Autodesk Inventor part; units mm, degrees
ref_plane "YZ Plane" through (0, 0, 0) normal (1, 0, 0) x (0, 1, 0)
ref_plane "XZ Plane" through (0, 0, 0) normal (0, 1, 0) x (-1, 0, 0)
ref_plane "XY Plane" through (0, 0, 0) normal (0, 0, 1) x (1, 0, 0)
sketch "Sketch1" plane through (0, 0, 0) normal (1, 0, 0) x (0, 1, 0)
  line L0 (0, 0) -> (44, 0)
  line L1 (44, 0) -> (44, 44)
  line L2 (44, 44) -> (0, 44)
  line L3 (0, 44) -> (0, 0)
  dimension "d2" = 44
extrude "Extrusion1" add sketch "Sketch1" along normal blind 12
sketch "Sketch2" plane through (12, 0, 0) normal (1, 0, 0) x (0, 0, -1)
  line L0 (-44, 44) -> (-44, 0)
  line L1 (0, 44) -> (-44, 44)
  point P0 (0, 0)
  point P1 (-5, 5)
  point P2 (-39, 5)
  point P3 (-39, 39)
  point P4 (-5, 39)
  dimension "d3" = 5
  dimension "d4" = 5
  dimension "d5" = 5
  dimension "d6" = 5
hole "Hole1" at (12, 5, 5) at (12, 5, 39) at (12, 39, 39) at (12, 39, 5) direction (-1, 0, 0) diameter 6 end through all
sketch "Sketch3" plane through (0, 44, 44) normal (0, 1, 0) x (1, 0, 0)
  line L0 (0, 0) -> (12, 0)
  point P0 (0, 44)
  point P1 (6, 22)
  dimension "d14" = 6
  dimension "d15" = 22
hole "Hole2" at (6, 44, 22) direction (0, -1, 0) diameter 6 end through all
sketch "Sketch4" plane through (0, 44, 44) normal (0, 1, 0) x (1, 0, 0)
  circle A0 centre (6, 22) radius 3
  line L0 (0, 44) -> (0, 0)
  line L1 (0, 0) -> (12, 0)
  line L2 (12, 44) -> (12, 0)
  line L3 (0, 44) -> (12, 44)
  circle A1 centre (6, 22) radius 3
  circle A2 centre (6, 22) radius 6
  line L4 (0, 44) -> (12, 44)
  line L5 (0, 0) -> (12, 0)
  line L6 (12, 44) -> (12, 0)
  line L7 (12, 0) -> (6, 0)
  line L8 (6, 0) -> (6, 44)
  line L9 (6, 44) -> (12, 44)
  line L10 (12, 44) -> (12, 0)
  point P0 (6, 28)
  point P1 (12, 22)
  point P2 (6, 16)
  point P3 (6, 0)
  dimension "d23" = 6
extrude "Extrusion2" cut sketch "Sketch4" against normal blind 50 contours L8 L3 L2 A2 | A2 L2 L1 L8
fillet "Fillet1" radius 5 2 edges at (6, 22, 28) (6, 22, 16)
properties part number "Piston Mount"
Verification items for the finished model (mm, model axes). A direction names the side the tool comes from. Coordinates: 2 decimals unless noted, no trailing zeros. Order: outer loops, then holes, each group sorted by start corner. A loop starts at its lowest first (then second) coordinate and runs counter-clockwise, first axis right, second up. Notation, with made-up numbers: (-17.5, 62) -> (16.5, 62) arc R26 cw to (16.5, 99) -> close; hole circle Ø10 at (56, -3.75). An arc over 180 degrees is marked (long way). Put each result on its own line as item: value. Start each with the question number.
1) Release check for a two-part mould opening along Y. For faces 1 (the cylindrical face through (3, 36, 5)), 2 (the flat face through (6, 22, 6)), 3 (the flat face through (2, 44, 22)) record: pulls with the +Y half, pulls with the -Y half, needs draft (parallel to the pull), parting line crosses it, or undercut.
2) Cross-section at A-A (y = 39). Enter the section's corners in (x, z), plus the area to 3 significant figures.
3) Cross-section at C-C (x = 5). Enter the section's corners in (y, z).
4) Cross-section at B-B (z = 22). Enter the section's corners in (x, y), plus the area to 3 significant figures.
5) Go/stop test with flat-tipped pins: pin 1 (4 mm diameter, centred on x = 6, z = 7, fed in from -Y); pin 2 (10 mm diameter, centred on y = 22, z = 4.5, fed in from +X). Record where each tip stops, or that it passes through.
6) Cross-section at D-D (y = 9.5). Enter the section's corners in (x, z).
7) Tool access check on faces 4 (the flat face through (6, 22, 38)), 5 (the flat face through (3, 22, 44)). Record the directions out of +Z, -Z, +X, -X, +Y, -Y that give a thin tool (end or side, any length) a straight path to the whole face; none if there is none.
8) Material ranges on L1, parallel to Y at x = 1.25, z = 39; L2, parallel to X at y = 24.5, z = 22; L3, parallel to Z at x = 3.4, y = 5, recorded low to high.
Geometry check:
1. face 1: undercut
1. face 2: needs draft
1. face 3: pulls with the +Y half
2. outline: (0, 0) -> (6, 0) -> (6, 2) -> (0, 2) -> close; (0, 8) -> (6, 8) -> (6, 12.2) arc R5 cw to (8.73, 16.66) arc R6 ccw to (8.73, 27.34) arc R5 cw to (6, 31.8) -> (6, 36) -> (0, 36) -> close; (0, 42) -> (6, 42) -> (6, 44) -> (0, 44) -> close; hole circle Ø6 at (6, 22)
2. area: 225 mm^2
3. outline: (0, 0) -> (44, 0) -> (44, 19.17) -> (0, 19.17) -> close; (0, 24.83) -> (44, 24.83) -> (44, 44) -> (0, 44) -> close; hole circle Ø6 at (5, 5); hole circle Ø6 at (5, 39); hole circle Ø6 at (39, 5); hole circle Ø6 at (39, 39)
4. outline: (0, 0) -> (3, 0) -> (3, 44) -> (0, 44) -> close; (9, 0) -> (12, 0) -> (12, 44) -> (9, 44) -> close
4. area: 264 mm^2
5. pin 1: stops at y = 0
5. pin 2: stops at x = 6
6. outline: (0, 0) -> (6, 0) -> (6, 12.2) arc R5 cw to (8.73, 16.66) arc R6 ccw to (8.73, 27.34) arc R5 cw to (6, 31.8) -> (6, 44) -> (0, 44) -> close; hole circle Ø6 at (6, 22)
7. face 4: +Z, +X, +Y, -Y
7. face 5: +Z, +X, -X, +Y, -Y
8. L1: y = 0 to 2, 8 to 36, 42 to 44
8. L2: x = 0 to 3, 9 to 12
8. L3: z = 0 to 2, 8 to 20.5, 23.5 to 36, 42 to 44
